For this review, take the finished solid that the model builds, in its own axes (mm). Face numbers are marked on the shaded views. A direction names the side the tool comes from. Give positions to 0.01 mm unless a question says otherwise; leave off trailing zeros. Write each loop counter-clockwise with the first axis right and the second up, starting at its lowest first coordinate (ties: lowest second). Pieces come first, ordered by that corner, then holes.
Q1. For line 1 (Y direction, x = 35, z = 24.6); line 2 (Z direction, x = 10, y = -8); line 3 (Y direction, x = 68, z = 8.25), list the stretches that pass through material, from the lowest coordinate up.
Q2. We need section B-B (x = 35). Write out the cut boundary in (y, z).
Q3. We need section C-C (z = 17.75). Write out the cut boundary in (x, y).
Q4. We need section A-A (y = 0). Write out the cut boundary in (x, z), then the cut area to 3 significant figures.
Q5. Machinability: for the marked faces 1, 2, 3, 4 and 5, which of the approach directions +Z, -Z, +X, -X, +Y, -Y give a long, thin tool a straight path to every point of the face, cutting with its end or side? Answer none if there is none.
Q6. Mouldability with a two-part tool opening along Y and no side actions: class the marked faces 6, 7 and 8 as released by +Y, released by -Y, zero draft, split by the parting line, or undercut.
Q7. Insertion check: P1, Ø12, axis at x = 9, z = 4, coming from the +Y side; P2, Ø4, axis at x = 23, y = -4.5, coming from the +Z side; P3, Ø9.5, axis at x = 35, y = 0, coming from the +Z side. Each pin has a flat end and moves straight along its axis. Give the tip position at first contact, or say it passes through.
Q8. We need section D-D (x = 67). Write out the cut boundary in (y, z).
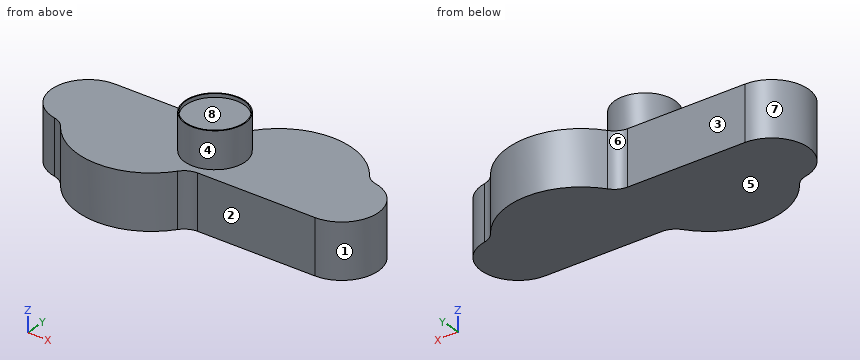
```python
from build123d import *

# Parameters (mm, degrees)
BOSS_EXTRUDE5_DEPTH = 15
SKETCH5_R           = 8.25
BOSS_EXTRUDE6_DEPTH = 10
SKETCH6_R           = 8
CUT_EXTRUDE2_DEPTH  = 1
FILLET3_R           = 5


with BuildPart() as part:
    # Sketch1 → Boss-Extrude5 (new body)
    with BuildSketch(Plane.XY):
        with BuildLine():
            Line((35, 10), (0, 10))
            ThreePointArc((0, 10), (-10, 0), (0, -10))
            Line((0, -10), (35, -10))
            Line((35, -10), (70, -10))
            ThreePointArc((70, -10), (80, 0), (70, 10))
            Line((70, 10), (35, 10))
        make_face()
        with BuildLine():
            ThreePointArc((70, 10), (52.5, 20.155644371), (35, 10))
            Line((35, 10), (70, 10))
        make_face()
        with BuildLine():
            Line((35, -10), (0, -10))
            ThreePointArc((0, -10), (17.5, -20.155644371), (35, -10))
        make_face()
    extrude(amount=BOSS_EXTRUDE5_DEPTH)

    # Sketch5 → Boss-Extrude6 (add)
    with BuildSketch(Plane.XY.offset(15)):
        with Locations((35, 0)):
            Circle(SKETCH5_R)
    extrude(amount=BOSS_EXTRUDE6_DEPTH)

    # Sketch6 → Cut-Extrude2 (cut)
    with BuildSketch(Plane.XY.offset(25)):
        with Locations((35, 0)):
            Circle(SKETCH6_R)
    extrude(amount=-CUT_EXTRUDE2_DEPTH, mode=Mode.SUBTRACT)

    # Fillet3
    fillet3_edges = [part.edges().sort_by_distance(p)[0] for p in [
        (35, -10, 7.5),
        (0, -10, 7.5),
        (35, 10, 7.5),
        (70, 10, 7.5),
    ]]
    fillet(fillet3_edges, radius=FILLET3_R)


solid = part.part
```
Computed:
1. line 1: y = -8.25 to -8, 8 to 8.25
1. line 2: z = 0 to 15
1. line 3: y = -10 to 12.88
2. outline: (-10.79, 0) - (10.79, 0) - (10.79, 15) - (8.25, 15) - (8.25, 25) - (8, 25) - (8, 24) - (-8, 24) - (-8, 25) - (-8.25, 25) - (-8.25, 15) - (-10.79, 15) - close
3. outline: circle Ø16.5 at (35, 0)
4. outline: (-10, 0) - (80, 0) - (80, 15) - (43.25, 15) - (43.25, 25) - (43, 25) - (43, 24) - (27, 24) - (27, 25) - (26.75, 25) - (26.75, 15) - (-10, 15) - close
4. area: 1,500 mm2
5. face 1: +Z, -Z, +X
5. face 2: +Z, -Z, +X, -Y
5. face 3: +Z, -Z, -X, +Y
5. face 4: +Z
5. face 5: -Z, +X, -X, +Y, -Y
6. face 6: released by +Y
6. face 7: split by the parting line
6. face 8: undercut
7. P1: stops at y = 10
7. P2: stops at z = 15
7. P3: stops at z = 24
8. outline: (-10, 0) - (14, 0) - (14, 15) - (-10, 15) - close
